Could you check a few things on this model? Use its own coordinates, in mm. Round coordinates to 2 decimals unless told otherwise and drop trailing zeros. Loops run counter-clockwise (first coordinate to the right, second up) from the corner with the lowest first, then second, coordinate; pieces in that order, holes last. Notation, with made-up numbers: M 24.5,82 L 65.5,82 A19 ccw 65.5,119 Z; hole C 56.25,-19 d3. An arc over 180 degrees is marked long. Return JSON: item names as keys, results as strings. Group by question number.
```python
from build123d import *

# Parameters (mm, degrees)
SKETCH_1_W          = 12
SKETCH_1_H          = 4
EXTRUDE_1_DEPTH     = 4
SKETCH_2_R          = 1
CUT_EXTRUDE_1_DEPTH = 11
SKETCH_3_R          = 1
CUT_EXTRUDE_2_DEPTH = 11


with BuildPart() as part:
    # 草圖1 → 填料-伸長1 (new body)
    with BuildSketch(Plane.XY):
        with Locations((-0.194141854, 1.08496732)):
            Rectangle(SKETCH_1_W, SKETCH_1_H)
    extrude(amount=EXTRUDE_1_DEPTH)

    # 草圖2 → 除料-伸長1 (cut)
    with BuildSketch(Plane.XZ.offset(0.91503268)):
        with Locations(Location((-4.194141854, 2, 0), (0, 0, 270))):
            Circle(SKETCH_2_R)
        with Locations(Location((3.805858146, 2, 0), (0, 0, 270))):
            Circle(SKETCH_2_R)
    extrude(amount=-CUT_EXTRUDE_1_DEPTH, mode=Mode.SUBTRACT)

    # 草圖3 → 除料-伸長2 (cut)
    with BuildSketch(Plane.XY.offset(4)):
        with Locations((-0.194141854, 1.08496732)):
            Circle(SKETCH_3_R)
    extrude(amount=-CUT_EXTRUDE_2_DEPTH, mode=Mode.SUBTRACT)


solid = part.part
```
1. If we section it at D-D, the plane y = 1.7: Please give me the cut outline in (x, z), then the cut area to 3 significant figures.
2. I need wall thicknesses on probe 1 along X at (y, z) = (-0.55, 2.55); probe 2 along X at (y, z) = (-0.55, 2.9); probe 3 along X at (y, z) = (1.3, 2.4). Which ranges of each line are inside material? Lowest first, please.
3. If we section it at A-A, the plane z = 1.8: Please give me the cut outline in (x, y), then the cut area to 3 significant figures.
4. If we section it at B-B, the plane y = 0.8: Please give me the cut outline in (x, z), then the cut area to 3 significant figures.
5. We'd pull the mould along X, two halves only. Please class faces 1 (the face through (-6.194, 1, 2)), 2 (the face through (0, 3.085, 2)), 3 (the face through (3.197, 1.057, 2.794)): +X half, -X half, draft (parallel to the pull), parting line (faces both ways), or undercut.
6. If we section it at C-C, the plane z = 0.3: Please give me the cut outline in (x, y), then the cut area to 3 significant figures.
Geometry results:
{
 "1": {"outline": "M -6.19,0 L -0.98,0 L -0.98,4 L -6.19,4 Z; M 0.59,0 L 5.81,0 L 5.81,4 L 0.59,4 Z; hole C -4.19,2 d2; hole C 3.81,2 d2", "area": "35.4 mm^2"},
 "2": {"probe 1": "-6.19 to -5.03, -3.36 to 2.97, 4.64 to 5.81", "probe 2": "-6.19 to -4.63, -3.76 to 3.37, 4.24 to 5.81", "probe 3": "-6.19 to -5.11, -3.28 to -1.17, 0.78 to 2.89, 4.72 to 5.81"},
 "3": {"outline": "M -6.19,-0.92 L -5.17,-0.92 L -5.17,3.08 L -6.19,3.08 Z; M -3.21,-0.92 L 2.83,-0.92 L 2.83,3.08 L -3.21,3.08 Z; M 4.79,-0.92 L 5.81,-0.92 L 5.81,3.08 L 4.79,3.08 Z; hole C -0.19,1.08 d2", "area": "29.2 mm^2"},
 "4": {"outline": "M -6.19,0 L -1.15,0 L -1.15,4 L -6.19,4 Z; M 0.76,0 L 5.81,0 L 5.81,4 L 0.76,4 Z; hole C -4.19,2 d2; hole C 3.81,2 d2", "area": "34.0 mm^2"},
 "5": {"face 1": "-X half", "face 2": "draft", "face 3": "undercut"},
 "6": {"outline": "M -6.19,-0.92 L 5.81,-0.92 L 5.81,3.08 L -6.19,3.08 Z; hole C -0.19,1.08 d2", "area": "44.9 mm^2"}
}
